For this review, take the finished solid that the model builds, in its own axes (mm). A direction names the side the tool comes from. Round coordinates to 2 decimals unless told otherwise and drop trailing zeros. Loops run counter-clockwise (first coordinate to the right, second up) from the corner with the lowest first, then second, coordinate; pieces in that order, holes last. Notation, with made-up numbers: (22, 79.5) -> (76, 79.5) arc R26 cw to (76, 100.5) -> close; hole circle Ø6 at (-8.75, -8.75). An arc over 180 degrees is marked (long way). Use one line per item in the form item = value. Start each with the question number.
from build123d import *

# Parameters (mm, degrees)
SKETCH_1_R          = 1.5
SKETCH_1_R_2        = 2
SKETCH_1_W          = 4.4
SKETCH_1_H          = 8.4
EXTRUDE_1_DEPTH     = 4
CUT_EXTRUDE_1_DEPTH = 10


with BuildPart() as part:
    # 草图1 → 凸台-拉伸1 (new body)
    with BuildSketch(Plane.XY):
        with BuildLine():
            Line((-6, 39), (-6, -39))
            Line((-6, -39), (245.772887801, -39))
            ThreePointArc((245.772887801, -39), (250.169785399, -38.08301996), (253.833616208, -35.484962093))
            Line((253.833616208, -35.484962093), (285.490974876, -1.392421989))
            ThreePointArc((285.490974876, -1.392421989), (287.669094365, 2.071844423), (288.430246468, 6.092540104))
            Line((288.430246468, 6.092540104), (288.430246468, 28))
            ThreePointArc((288.430246468, 28), (285.208421061, 35.778174593), (277.430246468, 39))
            Line((277.430246468, 39), (-6, 39))
        make_face()
        Circle(SKETCH_1_R, mode=Mode.SUBTRACT)
        with Locations((0, 26)):
            Circle(SKETCH_1_R, mode=Mode.SUBTRACT)
        with Locations((0, -26)):
            Circle(SKETCH_1_R, mode=Mode.SUBTRACT)
        with Locations((274, 35)):
            Circle(SKETCH_1_R_2, mode=Mode.SUBTRACT)
        with Locations((209, 35)):
            Circle(SKETCH_1_R_2, mode=Mode.SUBTRACT)
        with Locations((144, 35)):
            Circle(SKETCH_1_R_2, mode=Mode.SUBTRACT)
        with Locations((79, 35)):
            Circle(SKETCH_1_R_2, mode=Mode.SUBTRACT)
        with Locations((14, 35)):
            Circle(SKETCH_1_R_2, mode=Mode.SUBTRACT)
        with Locations((209, -35)):
            Circle(SKETCH_1_R_2, mode=Mode.SUBTRACT)
        with Locations((144, -35)):
            Circle(SKETCH_1_R_2, mode=Mode.SUBTRACT)
        with Locations((79, -35)):
            Circle(SKETCH_1_R_2, mode=Mode.SUBTRACT)
        with Locations((14, -35)):
            Circle(SKETCH_1_R_2, mode=Mode.SUBTRACT)
        with Locations((0, 13)):
            Rectangle(SKETCH_1_W, SKETCH_1_H, mode=Mode.SUBTRACT)
        with Locations((0, -13)):
            Rectangle(SKETCH_1_W, SKETCH_1_H, mode=Mode.SUBTRACT)
        Polygon((112.268773645, -27), (22, -27), (22, 21.606262732), align=None, mode=Mode.SUBTRACT)
        Polygon((45.731226355, 27), (136, 27), (136, -21.606262732), align=None, mode=Mode.SUBTRACT)
        Polygon((152, 18.345484713), (152, -18.345484713), (174.910889623, 0), align=None, mode=Mode.SUBTRACT)
        Polygon((236.71, -25), (236.71, 25), (264, 25), (264, 3.926902442), (237.139304875, -25), align=None, mode=Mode.SUBTRACT)
        with BuildLine():
            ThreePointArc((203.231094412, 19.08974359), (187.71, 0), (203.231094412, -19.08974359))
            ThreePointArc((203.231094412, -19.08974359), (207.21, -23.5), (211.188905588, -19.08974359))
            ThreePointArc((211.188905588, -19.08974359), (226.71, 0), (211.188905588, 19.08974359))
            ThreePointArc((211.188905588, 19.08974359), (207.21, 23.5), (203.231094412, 19.08974359))
        make_face(mode=Mode.SUBTRACT)
    extrude(amount=EXTRUDE_1_DEPTH)

    # 草图2 → 切除-拉伸1 (cut)
    with BuildSketch(Plane.XY.offset(4)):
        Polygon((279.349775131, 38.831223833), (279.349775131, -8.006021715), (315.852962883, -9.139766663), (310.030210466, 44.302513286), align=None)
    extrude(amount=-CUT_EXTRUDE_1_DEPTH, mode=Mode.SUBTRACT)


solid = part.part
Item 1: Take a section at A-A on x = 41.5. Give the boundary of the cut face in (y, z).
Item 2: Take a section at D-D on z = 1.9. Give the number of separate pieces and of enclosed holes in the cut face, plus the area to 3 significant figures.
Item 3: Take a section at B-B on x = 88. Give the boundary of the cut face in (y, z).
Item 4: For P1, Ø8, axis at x = 29.5, y = 18.5, coming from the -Z side; P2, Ø1.2, axis at x = 257, z = 1.5, coming from the -Y side, all flat-tipped, find the tip position at first contact; note any pin that passes through.
Item 5: Take a section at C-C on y = -13. Give the boundary of the cut face in (x, z), plus the area to 3 significant figures.
Item 6: Draft analysis for pull direction X (two halves, no side actions). For faces 3 (the flat face through (250.76, -10.33, 1.97)), 4 (the flat face through (135, -25, 0)), 5 (the flat face through (266.41, -21.94, 1.97)), state which applies: +X half, -X half, draft (parallel to the pull), parting line (faces both ways), or undercut.
Item 7: Wall thickness on line 1 (Y direction, x = 0, z = 1.8); line 2 (Y direction, x = 32.5, z = 0.2); line 3 (Y direction, x = 209, z = 1.9): over which ranges is each line inside the solid? List them lowest first.
Item 8: Machinability: for faces 1 (the flat face through (135, -25, 4)), 2 (the flat face through (163.62, 9.04, 1.97)), which of the approach directions +Z, -Z, +X, -X, +Y, -Y give a long, thin tool a straight path to every point of the face, cutting with its end or side? Answer none if there is none.
Results:
q1.outline = (-39, 0) -> (-27, 0) -> (-27, 4) -> (-39, 4) -> close; (11.11, 0) -> (39, 0) -> (39, 4) -> (11.11, 4) -> close
q2.separate_pieces = 1
q2.enclosed_holes = 19
q2.area = 14,600 mm2
q3.outline = (-39, 0) -> (-27, 0) -> (-27, 4) -> (-39, 4) -> close; (-13.93, 0) -> (4.24, 0) -> (4.24, 4) -> (-13.93, 4) -> close; (27, 0) -> (39, 0) -> (39, 4) -> (27, 4) -> close
q4.P1 = 0
q4.P2 = -32.72
q5.outline = (-6, 0) -> (-2.2, 0) -> (-2.2, 4) -> (-6, 4) -> close; (2.2, 0) -> (22, 0) -> (22, 4) -> (2.2, 4) -> close; (86.27, 0) -> (120.02, 0) -> (120.02, 4) -> (86.27, 4) -> close; (136, 0) -> (152, 0) -> (152, 4) -> (136, 4) -> close; (158.68, 0) -> (192.68, 0) -> (192.68, 4) -> (158.68, 4) -> close; (221.74, 0) -> (236.71, 0) -> (236.71, 4) -> (221.74, 4) -> close; (248.28, 0) -> (274.71, 0) -> (274.71, 4) -> (248.28, 4) -> close
q5.area = 595 mm2
q6.face_3 = undercut
q6.face_4 = draft
q6.face_5 = +X half
q7.line_1 = -39 to -27.5, -24.5 to -17.2, -8.8 to -1.5, 1.5 to 8.8, 17.2 to 24.5, 27.5 to 39
q7.line_2 = -39 to -27, 15.95 to 39
q7.line_3 = -39 to -37, -33 to -23.08, 23.08 to 33, 37 to 39
q8.face_1 = +Z, +X, -X, +Y, -Y
q8.face_2 = +Z, -Z
